from build123d import *

# Parameters (mm, degrees)
SKETCH1_R           = 2.5
SKETCH1_W           = 45
SKETCH1_H           = 264.057811959
SKETCH1_W_2         = 60
SKETCH1_H_2         = 100
BOSS_EXTRUDE1_DEPTH = 10
FILLET1_R           = 2


with BuildPart() as part:
    # Sketch1 → Boss-Extrude1 (new body)
    # profile 1 of 3: a face of its own
    with BuildSketch(Plane.XY):
        Polygon((77.5, -321.200669102), (32.5, -321.200669102), (25, -321.200669102), (25, -421.200669102), (85, -421.200669102), (85, -321.200669102), align=None)
        with Locations((42.094920328, -355.059007065)):
            Circle(SKETCH1_R, mode=Mode.SUBTRACT)
        with Locations((67.905079672, -387.342331139)):
            Circle(SKETCH1_R, mode=Mode.SUBTRACT)
    # profile 2 of 3: a face of its own
    with BuildSketch(Plane.XY):
        with Locations((55, -189.171763123)):
            Rectangle(SKETCH1_W, SKETCH1_H)
    # profile 3 of 3: a face of its own
    with BuildSketch(Plane.XY):
        with Locations((55, -7.142857143)):
            Rectangle(SKETCH1_W_2, SKETCH1_H_2)
        with Locations((42.094920328, 16.141662037)):
            Circle(SKETCH1_R, mode=Mode.SUBTRACT)
        with Locations((67.905079672, -16.141662037)):
            Circle(SKETCH1_R, mode=Mode.SUBTRACT)
    extrude(amount=BOSS_EXTRUDE1_DEPTH)

    # Fillet1
    fillet1_edges = [part.edges().sort_by_distance(p)[0] for p in [
        (25, -421.200669102, 5),
        (25, -321.200669102, 5),
        (32.5, -321.200669102, 5),
        (32.5, -57.142857143, 5),
        (25, -57.142857143, 5),
        (25, 42.857142857, 5),
        (85, 42.857142857, 5),
        (85, -57.142857143, 5),
        (77.5, -57.142857143, 5),
        (77.5, -321.200669102, 5),
        (85, -321.200669102, 5),
        (85, -421.200669102, 5),
    ]]
    fillet(fillet1_edges, radius=FILLET1_R)


solid = part.part
Source: CAD feature listing. Evaluate the final solid. Frame: model axes, mm. Round coordinates to 2 decimals unless told otherwise and drop trailing zeros. Write each loop counter-clockwise with the first axis right and the second up, starting at its lowest first coordinate (ties: lowest second). Pieces come first, ordered by that corner, then holes. Notation, with made-up numbers: M 31.5,20 L 90.5,20 A25 ccw 90.5,32 Z; hole C 11.5,83.25 d6. An arc over 180 degrees is marked long. One line per item, written item: value. Start each with the question number.
Item 1: Section query A-A (z = 6). Return the cut outline in (x, y), plus the area to 3 significant figures.
Item 2: Section query B-B (y = -101). Return the cut outline in (x, z), plus the area to 3 significant figures.
Item 3: Mould query, pull axis Y, two halves, no side actions, for faces 1 (the flat face through (32.5, -191, 5)), 2 (the flat face through (77.5, -191, 5)), 3 (the flat face through (55, -421.201, 5)), 4 (the flat face through (85, -8, 5)). Classes: pulls with the +Y half, pulls with the -Y half, needs draft (parallel to the pull), parting line crosses it, or undercut.
Item 4: Pin query (flat end, axial travel): pin 1 (3 mm diameter, centred on y = -145, z = 4.5, fed in from +X); pin 2 (3 mm diameter, centred on y = -215.5, z = 5.5, fed in from -X). Return the tip coordinate at first contact, or that it passes through.
Item 5: Ray query, L1, parallel to Y at x = 69, z = 6.25; L2, parallel to Y at x = 43, z = 2.5; L3, parallel to X at y = -225, z = 1.75. Return the intervals inside material, ascending. Write a range as from..to.
Result set:
1. outline: M 25,-419.2 A2 ccw 27,-421.2 L 83,-421.2 A2 ccw 85,-419.2 L 85,-323.2 A2 ccw 83,-321.2 L 79.5,-321.2 A2 cw 77.5,-319.2 L 77.5,-59.14 A2 cw 79.5,-57.14 L 83,-57.14 A2 ccw 85,-55.14 L 85,40.86 A2 ccw 83,42.86 L 27,42.86 A2 ccw 25,40.86 L 25,-55.14 A2 ccw 27,-57.14 L 30.5,-57.14 A2 cw 32.5,-59.14 L 32.5,-319.2 A2 cw 30.5,-321.2 L 27,-321.2 A2 ccw 25,-323.2 Z; hole C 42.09,-355.06 d5; hole C 42.09,16.14 d5; hole C 67.91,-387.34 d5; hole C 67.91,-16.14 d5
1. area: 23,800 mm²
2. outline: M 32.5,0 L 77.5,0 L 77.5,10 L 32.5,10 Z
2. area: 450 mm²
3. face 1: undercut
3. face 2: undercut
3. face 3: pulls with the -Y half
3. face 4: needs draft
4. pin 1: stops at x = 77.5
4. pin 2: stops at x = 32.5
5. L1: y = -421.2..-389.59, -385.09..-18.39, -13.89..42.86
5. L2: y = -421.2..-357.39, -352.73..13.81, 18.47..42.86
5. L3: x = 32.5..77.5
